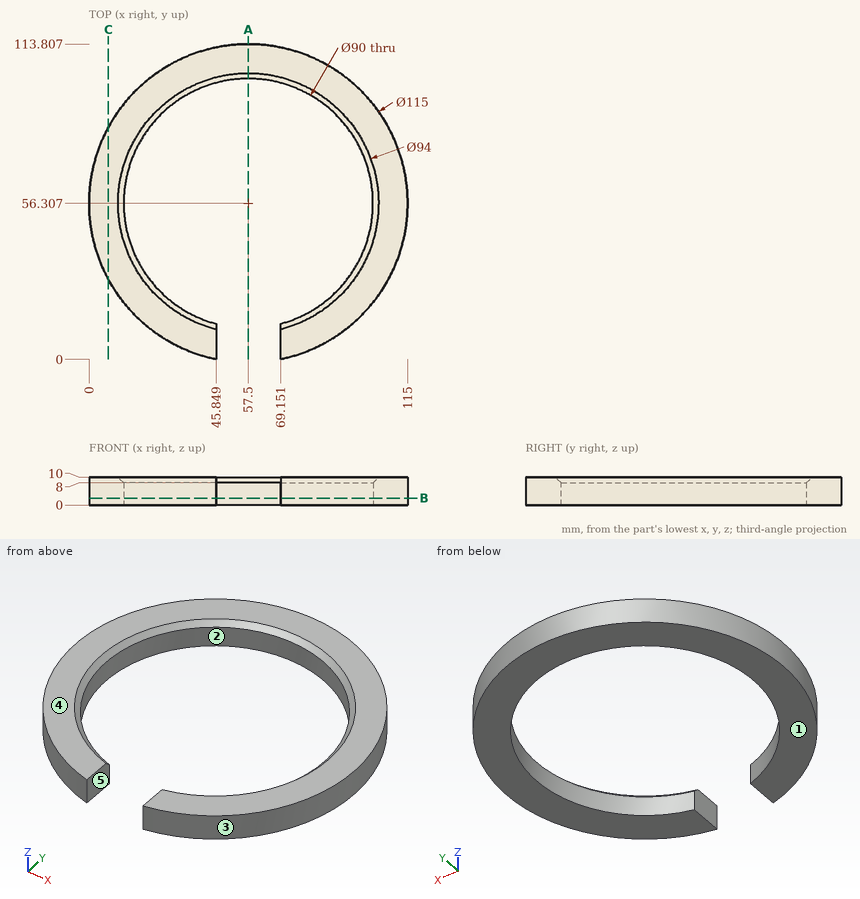
Geometry: see drawing. Coordinates: mm, zero at the bounding-box minimum. A direction names the side the tool comes from. Coordinates: 2 decimals unless noted, no trailing zeros. Write each loop counter-clockwise with the first axis right and the second up, starting at its lowest first coordinate (ties: lowest second). Pieces come first, ordered by that corner, then holes. Notation, with made-up numbers: M -31,-15.5 L 1,-15.5 A13 ccw 1,1.5 Z; hole C -12,35 d6. An arc over 180 degrees is marked long. Use CSV: the item, a comma, the result in double quotes. Start each with the question number.
1. Cut plane B-B on z = 2.5. Return the cut outline in (x, y), plus the area to 3 significant figures.
2. Cut plane A-A on x = 57.5. Return the cut outline in (y, z), plus the area to 3 significant figures.
3. Cut plane C-C on x = 7. Return the cut outline in (y, z).
4. Ray query, probe 1 along Y at (x, z) = (43.5, 2.75) (1 decimal); probe 2 along Y at (x, z) = (57.5, 4.75); probe 3 along Y at (x, z) = (17.5, 6.75) (1 decimal). Return the intervals inside material, ascending.
5. Reachability of the marked faces 4 and 5 from +Z, -Z, +X, -X, +Y, -Y: full face, straight path, thin tool, end or side. Return the list, or none.
6. First-contact query: P1, Ø1, axis at x = 28.5, z = 7.5, coming from the -Y side; P2, Ø5, axis at y = 9, z = 7, coming from the +X side (1 decimal); P3, Ø6, axis at y = 21, z = 3.5, coming from the +X side (1 decimal). Flat tips, straight axial feed; report the tip coordinate or a pass-through.
7. Mould query, pull axis X, two halves, no side actions, for the marked faces 1, 2 and 3. Classes: pulls with the +X half, pulls with the -X half, needs draft (parallel to the pull), parting line crosses it, or undercut.
Entries:
1,outline,"M 45.85,0 L 45.85,12.84 A45 cw long 69.15,12.84 L 69.15,0 A57.5 ccw long Z"
1,area,"3,730 mm²"
2,outline,"M 101.31,0 L 113.81,0 L 113.81,10 L 103.31,10 L 101.31,8 Z"
2,area,"123 mm²"
3,outline,"M 28.81,0 L 83.8,0 L 83.8,10 L 28.81,10 Z"
4,probe 1,"0.5 to 13.5, 99.1 to 112.1"
4,probe 2,"101.31 to 113.81"
4,probe 3,"15 to 35.7, 76.9 to 97.6"
5,face 4,"+Z, +X, -X, +Y, -Y"
5,face 5,"+Z, -Z, -Y"
6,P1,"y = 6.37"
6,P2,"x = 93.5"
6,P3,"x = 105.1"
7,face 1,"needs draft"
7,face 2,"undercut"
7,face 3,"parting line crosses it"
